Read the model definition and answer for the solid it produces. Units are mm, in the model's axes. A direction names the side the tool comes from. Give positions to 0.01 mm unless a question says otherwise; leave off trailing zeros. Write each loop counter-clockwise with the first axis right and the second up, starting at its lowest first coordinate (ties: lowest second). Pieces come first, ordered by that corner, then holes. Notation, with made-up numbers: (54, -28.75) - (80, -28.75) arc R23 cw to (80, -14.75) - close; hole circle Ø3 at (75, 12.25). An arc over 180 degrees is marked (long way). Answer as a JSON object with one key per item and string values. Group by question number.
```python
from build123d import *

# Parameters (mm, degrees)
PAD002_DEPTH  = 1.5
PAD003_DEPTH  = 0.5
SKETCH005_R   = 1.025
PAD004_DEPTH  = 4.6
SKETCH006_R   = 2.1
POCKET_DEPTH  = 2
SKETCH008_R   = 2
SKETCH008_R_2 = 1.6
PAD005_DEPTH  = 3
PAD014_DEPTH  = 1.5


with BuildPart() as part:
    # Sketch003 → Pad002 (new body)
    with BuildSketch(Plane.XY.offset(6)):
        with BuildLine():
            Line((-29.25, 12.75), (29.25, 12.75))
            ThreePointArc((33, 9), (31.9016504294, 11.6516504294), (29.25, 12.75))
            Line((33, 9), (33, -9))
            ThreePointArc((29.25, -12.75), (31.9016504295, -11.6516504294), (33, -9))
            Line((29.25, -12.75), (-29.25, -12.75))
            ThreePointArc((-33, -9), (-31.9016504294, -11.6516504295), (-29.25, -12.75))
            Line((-33, -9), (-33, 9))
            ThreePointArc((-29.25, 12.75), (-31.9016504294, 11.6516504294), (-33, 9))
        make_face()
    extrude(amount=PAD002_DEPTH)

    # Sketch004 → Pad003 (new body)
    with BuildSketch(Plane(origin=(0, 0, 6), x_dir=(1, 0, 0), z_dir=(0, 0, -1))):
        with BuildLine():
            Line((-29.05, 11.05), (29.05, 11.05))
            ThreePointArc((31.3, 8.8), (30.6409902577, 10.3909902577), (29.05, 11.05))
            Line((31.3, 8.8), (31.3, -8.8))
            ThreePointArc((29.05, -11.05), (30.6409902577, -10.3909902577), (31.3, -8.8))
            Line((29.05, -11.05), (-29.05, -11.05))
            ThreePointArc((-31.3, -8.8), (-30.6409902577, -10.3909902577), (-29.05, -11.05))
            Line((-31.3, -8.8), (-31.3, 8.8))
            ThreePointArc((-29.05, 11.05), (-30.6409902577, 10.3909902577), (-31.3, 8.8))
        make_face()
    extrude(amount=PAD003_DEPTH)

    # Sketch005 → Pad004 (new body)
    with BuildSketch(Plane(origin=(0, 0, 5.5), x_dir=(1, 0, 0), z_dir=(0, 0, -1))):
        with BuildLine():
            Line((-25.75, -9), (-25.75, -11.05))
            Line((-25.75, -11.05), (-29.05, -11.05))
            ThreePointArc((-31.3, -8.8), (-30.6409902577, -10.3909902577), (-29.05, -11.05))
            Line((-31.3, -6.75), (-31.3, -8.8))
            Line((-27.9999999649, -6.75), (-31.3, -6.75))
            ThreePointArc((-25.75, -9.0000000351), (-26.4090097175, -7.4090097671), (-27.9999999649, -6.75))
        make_face()
        with Locations((-28, -9)):
            Circle(SKETCH005_R, mode=Mode.SUBTRACT)
        with BuildLine():
            ThreePointArc((25.75, 9), (26.4090097423, 7.4090097423), (28, 6.75))
            Line((28, 6.75), (31.3, 6.75))
            Line((31.3, 8.8), (31.3, 6.75))
            ThreePointArc((31.3, 8.8), (30.6409902577, 10.3909902577), (29.05, 11.05))
            Line((29.05, 11.05), (25.75, 11.05))
            Line((25.75, 11.05), (25.75, 9))
        make_face()
        with Locations((28, 9)):
            Circle(SKETCH005_R, mode=Mode.SUBTRACT)
    extrude(amount=PAD004_DEPTH)

    # Sketch006 → Pocket (cut)
    with BuildSketch(Plane.XY.offset(7.5)):
        with Locations((-23, -7)):
            Circle(SKETCH006_R)
        with BuildLine():
            ThreePointArc((-24.3288922086, 3.1089076939), (-23.0026761128, 2.400002238), (-21.6740960519, 3.1044673539))
            ThreePointArc((-21.5638430432, 3.2946963807), (-21.7108688116, 3.2528448762), (-21.6740960519, 3.1044673539))
            ThreePointArc((-21.5638430432, 3.2946963807), (-21.6130238799, 4.7976824194), (-22.8873953748, 5.5960326433))
            ThreePointArc((-23.1072650483, 5.5964003913), (-22.9975078699, 5.4899979159), (-22.8873953748, 5.5960326433))
            ThreePointArc((-23.1072650483, 5.5964003913), (-24.3843000035, 4.8023175806), (-24.4385082583, 3.2995044678))
            ThreePointArc((-24.3288922086, 3.1089076939), (-24.2916233116, 3.2571613762), (-24.4385082583, 3.2995044678))
        make_face()
    extrude(amount=-POCKET_DEPTH, mode=Mode.SUBTRACT)

    # Sketch008 → Pad005 (new body)
    with BuildSketch(Plane(origin=(0, 0, 5.5), x_dir=(1, 0, 0), z_dir=(0, 0, -1))):
        with Locations((-23, -4)):
            Circle(SKETCH008_R)
        with Locations((-23, -4)):
            Circle(SKETCH008_R_2, mode=Mode.SUBTRACT)
    extrude(amount=PAD005_DEPTH)

    # Sketch023 → Pad014 (new body)
    with BuildSketch(Plane(origin=(0, -11.05, 6), x_dir=(1, 0, 0), z_dir=(0, -1, 0))):
        with BuildLine():
            Line((11.5, 0), (18.5, 0))
            Line((18.5, 0), (18.5, -2.8))
            Line((18.5, -2.8), (17.6, -2.8))
            ThreePointArc((17.6, -2.8000000001), (15, -0.2000000001), (12.4, -2.8))
            Line((12.4, -2.8), (11.5, -2.8))
            Line((11.5, -2.8), (11.5, 0))
        make_face()
    extrude(amount=PAD014_DEPTH)


solid = part.part
```
1) Find section D-D, the plane y = -0.5. Write down the section's boundary in (x, z).
2) Find section A-A, the plane z = 1.75. Write down the section's boundary in (x, y) (3 decimals).
3) For a pull along X with two mould halves and no side action, classify faces 1 (the flat face through (28, -9, 5.5)), 2 (the flat face through (0, -12.75, 7)), 3 (the cylindrical face through (-30.66, 10.37, 3.49)) as released by +X, released by -X, zero draft, split by the parting line, or undercut.
4) Which of the six approach directions +Z, -Z, +X, -X, +Y, -Y give full straight-line access (tool end or side, diameter ignored) to faces 4 (the flat face through (-28, 9, 5.5)), 5 (the cylindrical face through (26.39, -7.43, 3.23)), 6 (the flat face through (11.5, -12, 5))?
5) Find the intervals of material crossed by line 1 (Y direction, x = -23, z = 5.9); line 2 (Y direction, x = -23, z = 6.3); line 3 (Y direction, x = -23, z = 4.45), in increasing order. Write a range as [from, to].
6) Find section B-B, the plane y = 4. Write down the section's boundary in (x, z), and give its area (3 significant figures).
7) Find section C-C, the plane z = 4.25. Write down the section's boundary in (x, y) (3 decimals).
8) Flat-ended cylindrical pins translate along their axes: pin 1 Ø0.7 at (x, z) = (12, 4.5) entering from +Y; pin 2 Ø4 at (x, y) = (-23, -7) entering from +Z; pin 3 Ø1.5 at (x, z) = (-20.5, 3) entering from +Y; pin 4 Ø1.6 at (x, y) = (28.5, -8.5) entering from -Z. Find the tip coordinate at first contact, or state that the pin passes through.
Values follow:
{
 "1": {"outline": "(-33, 6) - (-31.3, 6) - (-31.3, 5.5) - (31.3, 5.5) - (31.3, 6) - (33, 6) - (33, 7.5) - (-33, 7.5) - close"},
 "2": {"outline": "(-31.3, 6.75) - (-28, 6.75) arc R2.25 ccw to (-25.75, 9) - (-25.75, 11.05) - (-29.05, 11.05) arc R2.25 ccw to (-31.3, 8.8) - close; (25.75, -11.05) - (29.05, -11.05) arc R2.25 ccw to (31.3, -8.8) - (31.3, -6.75) - (28, -6.75) arc R2.25 ccw to (25.75, -9) - close; hole circle Ø2.05 at (-28, 9); hole circle Ø2.05 at (28, -9)"},
 "3": {"face 1": "undercut", "face 2": "zero draft", "face 3": "released by -X"},
 "4": {"face 4": "-Z", "face 5": "-Z, -X, +Y", "face 6": "-Z, -X, -Y"},
 "5": {"line 1": "y = [-11.05, -9.1], [-4.9, 2.4], [5.49, 11.05]", "line 2": "y = [-12.75, -9.1], [-4.9, 2.4], [5.49, 12.75]", "line 3": "y = [2, 2.4], [5.6, 6]"},
 "6": {"outline": "(-33, 6) - (-31.3, 6) - (-31.3, 5.5) - (-25, 5.5) - (-25, 2.5) - (-24.6, 2.5) - (-24.6, 7.5) - (-33, 7.5) - close; (-21.4, 2.5) - (-21, 2.5) - (-21, 5.5) - (31.3, 5.5) - (31.3, 6) - (33, 6) - (33, 7.5) - (-21.4, 7.5) - close", "area": "126 mm2"},
 "7": {"outline": "(-31.3, 6.75) - (-28, 6.75) arc R2.25 ccw to (-25.75, 9) - (-25.75, 11.05) - (-29.05, 11.05) arc R2.25 ccw to (-31.3, 8.8) - close; circle Ø4 at (-23, 4); (11.5, -12.55) - (12.621, -12.55) - (12.621, -11.05) - (11.5, -11.05) - close; (17.379, -12.55) - (18.5, -12.55) - (18.5, -11.05) - (17.379, -11.05) - close; (25.75, -11.05) - (29.05, -11.05) arc R2.25 ccw to (31.3, -8.8) - (31.3, -6.75) - (28, -6.75) arc R2.25 ccw to (25.75, -9) - close; hole circle Ø2.05 at (-28, 9); hole circle Ø3.2 at (-23, 4); hole circle Ø2.05 at (28, -9)"},
 "8": {"pin 1": "stops at y = -11.05", "pin 2": "passes through", "pin 3": "stops at y = 4.97", "pin 4": "stops at z = 0.9"}
}
